```python
from build123d import *

# Parameters (mm, degrees)
ESBO_O2_W                = 45
ESBO_O2_H                = 65
RESSALTO_EXTRUS_O2_DEPTH = 10
ESBO_O3_R                = 4.7625
CORTE_EXTRUS_O1_DEPTH    = 162.549920911
FURO_COM_FOLGA_DE_M31_D  = 3.4
ESBO_O6_R                = 3.75
CORTE_EXTRUS_O2_DEPTH    = 2.45


with BuildPart() as part:
    # Esboço2 → Ressalto-extrusão2 (new body)
    with BuildSketch(Plane.XY):
        with Locations((-19.282851211, 123.232367513)):
            Rectangle(ESBO_O2_W, ESBO_O2_H)
    extrude(amount=-RESSALTO_EXTRUS_O2_DEPTH)

    # Esboço3 → Corte-extrusão1 (cut, through all)
    with BuildSketch(Plane.XY):
        with Locations((-19.282851211, 136.502367513)):
            Circle(ESBO_O3_R)
        with Locations((-19.282851211, 110.732367513)):
            Circle(ESBO_O3_R)
    extrude(amount=-CORTE_EXTRUS_O1_DEPTH, mode=Mode.SUBTRACT)

    # Furo com folga de M31 (through all)
    with Locations(Plane(origin=(0.160463456, 1.173491391, -10), x_dir=(-1, 0, 0), z_dir=(0, 0, -1))):
        with Locations((19.443314667, 93.558876122), (19.443314667, 150.558876122), (0.943314667, 122.058876122), (37.943314667, 122.058876122)):
            Hole(FURO_COM_FOLGA_DE_M31_D / 2)

    # Esboço6 → Corte-extrusão2 (cut)
    with BuildSketch(Plane(origin=(0, 0, -10), x_dir=(-1, 0, 0), z_dir=(0, 0, -1))):
        with Locations((0.782851211, 123.232367513)):
            Circle(ESBO_O6_R)
    extrude(amount=-CORTE_EXTRUS_O2_DEPTH, mode=Mode.SUBTRACT)


solid = part.part
```
For this review, take the finished solid that the model builds, in its own axes (mm). A direction names the side the tool comes from. Round coordinates to 2 decimals unless told otherwise and drop trailing zeros. Write each loop counter-clockwise with the first axis right and the second up, starting at its lowest first coordinate (ties: lowest second). Pieces come first, ordered by that corner, then holes.
1) Machinability: for faces 1 (the face through (0.1, 121.6, -7.55)), 2 (the face through (-38.151, 121.573, -4.93)), which of the approach directions +Z, -Z, +X, -X, +Y, -Y give a long, thin tool a straight path to every point of the face, cutting with its end or side? Answer none if there is none.
Answer below:
face 1: -Z
face 2: +Z, -Z
2) Take a section at B-B on z = -4.5. Give the boundary of the cut face in (x, y) (1 decimal), then the cut area to 3 significant figures.
Answer below:
outline: (-41.8, 90.7) - (3.2, 90.7) - (3.2, 155.7) - (-41.8, 155.7) - close; hole circle Ø3.4 at (-37.8, 123.2); hole circle Ø9.5 at (-19.3, 110.7); hole circle Ø9.5 at (-19.3, 136.5); hole circle Ø3.4 at (-19.3, 94.7); hole circle Ø3.4 at (-19.3, 151.7); hole circle Ø3.4 at (-0.8, 123.2)
area: 2,750 mm2
3) Take a section at C-C on y = 134. Give the boundary of the cut face in (x, z), then the cut area to 3 significant figures.
Answer below:
outline: (-41.78, -10) - (-23.33, -10) - (-23.33, 0) - (-41.78, 0) - close; (-15.23, -10) - (3.22, -10) - (3.22, 0) - (-15.23, 0) - close
area: 369 mm2
4) Insertion check: pin 1 Ø7.5 at (x, y) = (-19.28, 136.5) entering from -Z. The pin has a flat end and moves straight along its axis. Give the tip position at first contact, or say it passes through.
Answer below:
pin 1: passes through
5) Take a section at A-A on y = 151. Give the boundary of the cut face in (x, z), then the cut area to 3 significant figures.
Answer below:
outline: (-41.78, -10) - (-20.82, -10) - (-20.82, 0) - (-41.78, 0) - close; (-17.75, -10) - (3.22, -10) - (3.22, 0) - (-17.75, 0) - close
area: 419 mm2
6) Mouldability with a two-part tool opening along X and no side actions: class faces 3 (the face through (3.217, 123, -5)), 4 (the face through (-19.903, 115.454, -4.93)), 5 (the face through (-20, 155.732, -5)) as +X half, -X half, draft (parallel to the pull), parting line (faces both ways), or undercut.
Answer below:
face 3: +X half
face 4: undercut
face 5: draft
7) For line 1 along X through (y, z) = (122, -2); line 2 along Y through (x, z) = (-22.5, -4.25); line 3 along Y through (x, z) = (-38.5, -3.5), list the stretches that pass through material, from the lowest coordinate up.
Answer below:
line 1: x = -41.78 to -38.95, -36.61 to -1.95, 0.39 to 3.22
line 2: y = 90.73 to 107.22, 114.24 to 132.99, 140.01 to 155.73
line 3: y = 90.73 to 121.69, 124.77 to 155.73
